Geometry check sheet. Reference: the model listing, model coordinates, mm. Face numbers are marked on the shaded views. A direction names the side the tool comes from. Coordinates: 2 decimals unless noted, no trailing zeros. Write each loop counter-clockwise with the first axis right and the second up, starting at its lowest first coordinate (ties: lowest second). Pieces come first, ordered by that corner, then holes.
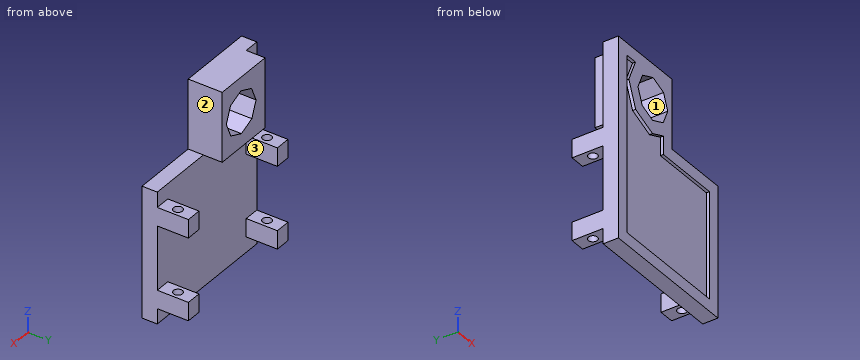
Autodesk Inventor part; units mm, degrees
ref_plane "YZ Plane" through (0, 0, 0) normal (1, 0, 0) x (0, 1, 0)
ref_plane "XZ Plane" through (0, 0, 0) normal (0, 1, 0) x (-1, 0, 0)
ref_plane "XY Plane" through (0, 0, 0) normal (0, 0, 1) x (1, 0, 0)
sketch "Sketch1" plane through (0, 0, 0) normal (0, 1, 0) x (-1, 0, 0)
  line L0 (10.0298, 10.8298) -> (-22.0758, 10.8298)
  line L1 (-22.0758, 10.8298) -> (-22.0758, -18.1453)
  line L2 (-22.0758, -18.1453) -> (10.0298, -18.1453)
  line L3 (10.0298, -18.1453) -> (10.0298, 10.8298)
  line L4 (10.0298, 10.8298) -> (0.708, 10.8298)
  line L5 (10.0298, 4.4798) -> (10.0298, 10.8298)
  line L6 (10.0298, -18.1453) -> (0.708, -18.1453)
  line L7 (10.0298, -11.954) -> (10.0298, -18.1453)
  line L8 (-22.0758, 4.4798) -> (-22.0758, -11.954)
  line L9 (-4.274, -9.9621) -> (-10.5532, -12.6713)
  line L10 (-10.5532, -12.6713) -> (-16.9089, -10.147)
  line L11 (-16.9089, -10.147) -> (-19.6181, -3.8679)
  line L12 (-19.6181, -3.8679) -> (-17.0938, 2.4878)
  line L13 (-17.0938, 2.4878) -> (-10.8147, 5.1971)
  line L14 (-10.8147, 5.1971) -> (-4.459, 2.6728)
  line L15 (-4.459, 2.6728) -> (-1.7498, -3.6063)
  line L16 (-1.7498, -3.6063) -> (-4.274, -9.9621)
  point P0 (0, 0)
  point P1 (-10.6839, -3.7371)
  dimension "d0" = 28.975
  dimension "d1" = 32.1056
extrude "Extrusion1" add sketch "Sketch1" along normal blind 14.224
sketch "Sketch2" plane through (0, 0, 0) normal (0, -1, 0) x (1, 0, 0)
  line L0 (-10.0298, -18.1453) -> (-10.0298, 10.8298)
  line L1 (-10.0298, -18.1453) -> (49.7745, -18.1453)
  line L2 (49.7745, -18.1453) -> (49.7745, -24.4953)
  line L3 (49.7745, -24.4953) -> (-10.0298, -24.4953)
  line L4 (-10.0298, -24.4953) -> (-10.0298, -18.1453)
  line L5 (-10.0298, -24.4953) -> (49.7745, -24.4953)
  line L6 (49.7745, -24.4953) -> (49.7745, -72.7553)
  line L7 (49.7745, -72.7553) -> (-10.0298, -72.7553)
  line L8 (-10.0298, -72.7553) -> (-10.0298, -24.4953)
  line L9 (-10.0298, -24.4953) -> (-3.6798, -24.4953)
  line L10 (-3.6798, -24.4953) -> (-3.6798, -32.1153)
  line L11 (-3.6798, -32.1153) -> (-10.0298, -32.1153)
  line L12 (-10.0298, -32.1153) -> (-10.0298, -24.4953)
  line L13 (49.7745, -24.4953) -> (43.4245, -24.4953)
  line L14 (43.4245, -24.4953) -> (43.4245, -32.1153)
  line L15 (43.4245, -32.1153) -> (49.7745, -32.1153)
  line L16 (49.7745, -32.1153) -> (49.7745, -24.4953)
  line L17 (49.7745, -72.7553) -> (-10.0298, -72.7553)
  line L18 (-10.0298, -72.7553) -> (-10.0298, -66.4053)
  line L19 (-10.0298, -66.4053) -> (49.7745, -66.4053)
  line L20 (49.7745, -66.4053) -> (49.7745, -72.7553)
  line L21 (-10.0298, -66.4053) -> (-3.6798, -66.4053)
  line L22 (-3.6798, -66.4053) -> (-3.6798, -58.7853)
  line L23 (-3.6798, -58.7853) -> (-10.0298, -58.7853)
  line L24 (-10.0298, -58.7853) -> (-10.0298, -66.4053)
  line L25 (49.7745, -66.4053) -> (43.4245, -66.4053)
  line L26 (43.4245, -66.4053) -> (43.4245, -58.7853)
  line L27 (43.4245, -58.7853) -> (49.7745, -58.7853)
  line L28 (49.7745, -58.7853) -> (49.7745, -66.4053)
  point P0 (0, 0)
  dimension "d8" = 59.8043
  dimension "d9" = 6.35
  dimension "d10" = 48.26
  dimension "d11" = 6.35
  dimension "d12" = 7.62
  dimension "d13" = 6.35
  dimension "d14" = 6.35
  dimension "d15" = 6.35
  dimension "d16" = 7.62
extrude "Extrusion2" add sketch "Sketch2" against normal blind 6.35
sketch "Sketch3" plane through (0, 6.35, 0) normal (0, 1, 0) x (1, 0, 0)
  line L0 (-10.0298, -10.8298) -> (-10.0298, 72.7553)
  line L1 (49.7745, 18.1453) -> (49.7745, 72.7553)
  line L2 (-10.0298, 72.7553) -> (49.7745, 72.7553)
  line L3 (49.7745, 72.7553) -> (49.7745, 66.4053)
  line L4 (49.7745, 66.4053) -> (-10.0298, 66.4053)
  line L5 (-10.0298, 66.4053) -> (-10.0298, 72.7553)
  line L6 (-10.0298, 66.4053) -> (-3.6798, 66.4053)
  line L7 (-3.6798, 66.4053) -> (-3.6798, 58.7853)
  line L8 (-3.6798, 58.7853) -> (-10.0298, 58.7853)
  line L9 (-10.0298, 58.7853) -> (-10.0298, 66.4053)
  line L10 (49.7745, 66.4053) -> (43.4245, 66.4053)
  line L11 (43.4245, 66.4053) -> (43.4245, 58.7853)
  line L12 (43.4245, 58.7853) -> (49.7745, 58.7853)
  line L13 (49.7745, 58.7853) -> (49.7745, 66.4053)
  line L14 (22.0758, 18.1453) -> (-10.0298, 18.1453)
  line L15 (-10.0298, 18.1453) -> (-3.6798, 18.1453)
  line L16 (49.7745, 18.1453) -> (43.4245, 18.1453)
  line L17 (-10.0298, 18.1453) -> (49.7745, 18.1453)
  line L18 (49.7745, 24.4953) -> (-10.0298, 24.4953)
  line L19 (-10.0298, 24.4953) -> (-10.0298, 18.1453)
  line L20 (-10.0298, 24.4953) -> (-3.6798, 24.4953)
  line L21 (-3.6798, 24.4953) -> (-3.6798, 32.1487)
  line L22 (-3.6798, 32.1487) -> (-10.0298, 32.1487)
  line L23 (-10.0298, 32.1487) -> (-10.0298, 24.4953)
  line L24 (49.7745, 24.4953) -> (43.4245, 24.4953)
  line L25 (43.4245, 24.4953) -> (43.4245, 32.1487)
  line L26 (43.4245, 32.1487) -> (49.7745, 32.1487)
  line L27 (49.7745, 32.1487) -> (49.7745, 24.4953)
  point P0 (0, 0)
  dimension "d19" = 6.35
  dimension "d20" = 6.35
  dimension "d21" = 7.62
  dimension "d22" = 6.35
  dimension "d23" = 7.62
  dimension "d26" = 6.35
extrude "Extrusion3" add sketch "Sketch3" along normal blind 13.0048 contours L0 L22 L21 L18 | L0 L4 L7 L8 | L25 L26 L1 L18 | L4 L1 L12 L11
sketch "Sketch4" plane through (-10.0298, 0, 10.8298) normal (0, 0, 1) x (1, 0, 0)
  line L0 (32.1056, 14.224) -> (0, 14.224)
  line L1 (6.35, 6.35) -> (6.35, 19.3548)
  line L2 (0, 14.224) -> (6.35, 14.224)
  line L3 (6.35, 14.224) -> (6.35, 6.35)
  line L4 (6.35, 6.35) -> (0, 6.35)
  line L5 (0, 6.35) -> (0, 14.224)
  point P0 (10.0298, 0)
extrude "Extrusion4" cut sketch "Sketch4" along normal mid plane 64.7827
sketch "Sketch5" plane through (-3.6798, 6.35, -66.4053) normal (0, 0, -1) x (-1, 0, 0)
  line L0 (6.35, 13.0048) -> (0, 0)
  line L1 (0, 0) -> (0, 13.0048)
  line L2 (0, 0) -> (0, 13.0048)
  line L3 (0, 0) -> (6.35, 0)
  line L4 (0, 13.0048) -> (6.35, 0)
  line L5 (-53.4543, 0) -> (-53.4543, 13.0048)
  line L6 (-53.4543, 13.0048) -> (-47.2741, 0)
  line L7 (-47.2741, 13.0048) -> (-53.4543, 0)
  circle A0 centre (3.175, 6.5024) radius 1.8796
  circle A1 centre (-50.3642, 6.5024) radius 1.8796
  point P0 (-3.6798, -6.35)
  dimension "d31" = 3.7592
  dimension "d32" = 3.7592
extrude "Extrusion5" cut sketch "Sketch5" along normal mid plane 183.8452 contours A0 L4 L0 | L0 L4 A0 | L4 A0 L0 | L0 A0 L4 | A1 L6 L7 | L7 L6 A1 | A1 L7 L6 | L7 A1 L6
shell "Shell1" thickness 5.08 removed faces 1 at (20.6069, 0, -54.5519)
properties part number "leftside"
1. Thickness scan on line 1 along Z through (x, y) = (-1.5, 10.5); line 2 along Z through (x, y) = (-8, 17); line 3 along X through (y, z) = (7.25, -27). Record the ranges inside material, lowest first.
Computed values:
line 1: z = -18.15 to 10.83
line 2: z = -66.41 to -58.79, -32.15 to -24.5
line 3: x = -10.03 to -3.68, 43.42 to 49.77
2. Gauge pin test, flat ends, axial feed: pin 1 Ø7.5 at (x, z) = (3.5, -7) entering from +Y; pin 2 Ø3 at (x, y) = (41.5, 3.5) entering from +Z; pin 3 Ø8 at (y, z) = (10.5, -1.5) entering from +X. Record the tip position at first contact, or that the pin passes through.
Computed values:
pin 1: stops at y = 14.22
pin 2: stops at z = -18.15
pin 3: stops at x = 22.08
3. Access from +Z, -Z, +X, -X, +Y, -Y to the whole of each face (thin tool, end or side, straight path). Record for the marked faces 1, 2 and 3.
Computed values:
face 1: +Y, -Y
face 2: +Z, +X, +Y, -Y
face 3: -Z, +Y
4. Sectioned sample at D-D, the plane z = -42. Record the boundary of the cut face in (x, y).
Computed values:
outline: (-10.03, 0) - (-4.95, 0) - (-4.95, 1.27) - (44.69, 1.27) - (44.69, 0) - (49.77, 0) - (49.77, 6.35) - (-10.03, 6.35) - close
5. Sectioned sample at A-A, the plane y = 2.5. Record the boundary of the cut face in (x, z).
Computed values:
outline: (-10.03, -72.76) - (49.77, -72.76) - (49.77, -18.15) - (22.08, -18.15) - (22.08, 10.83) - (-10.03, 10.83) - close; hole (1.75, -3.61) - (4.27, -9.96) - (10.55, -12.67) - (16.91, -10.15) - (19.62, -3.87) - (17.09, 2.49) - (10.81, 5.2) - (4.46, 2.67) - close
6. Sectioned sample at B-B, the plane x = 46. Record the boundary of the cut face in (y, z).
Computed values:
outline: (0, -72.76) - (6.35, -72.76) - (6.35, -66.41) - (11.1, -66.41) - (11.1, -58.79) - (6.35, -58.79) - (6.35, -32.15) - (11.1, -32.15) - (11.1, -24.5) - (6.35, -24.5) - (6.35, -18.15) - (0, -18.15) - close; (14.6, -66.41) - (19.35, -66.41) - (19.35, -58.79) - (14.6, -58.79) - close; (14.6, -32.15) - (19.35, -32.15) - (19.35, -24.5) - (14.6, -24.5) - close
7. Sectioned sample at C-C, the plane y = 15.75. Record the boundary of the cut face in (x, z).
Computed values:
outline: (-10.03, -66.41) - (-3.68, -66.41) - (-3.68, -58.79) - (-10.03, -58.79) - close; (-10.03, -32.15) - (-3.68, -32.15) - (-3.68, -24.5) - (-10.03, -24.5) - close; (43.42, -66.41) - (49.77, -66.41) - (49.77, -58.79) - (43.42, -58.79) - close; (43.42, -32.15) - (49.77, -32.15) - (49.77, -24.5) - (43.42, -24.5) - close
